The listing builds one solid part. Answer for the finished solid, in the listing's coordinates (mm). A direction names the side the tool comes from. Give positions to 0.01 mm unless a question says otherwise; leave off trailing zeros. Write each loop counter-clockwise with the first axis right and the second up, starting at its lowest first coordinate (ties: lowest second). Pieces come first, ordered by that corner, then holes. Notation, with made-up numbers: (14.25, -37) - (39.25, -37) arc R16 ccw to (39.25, -28) - close; hole circle Ø8 at (36.5, -29). An arc over 180 degrees is marked (long way). Use a Markdown table: item, result. Add a question column.
from build123d import *

# Parameters (mm, degrees)
SKETCH1_R              = 1.5
BOSS_EXTRUDE1_DEPTH    = 3.6
FILLET1_R              = 1.5
LPATTERN2_COUNT        = 6
LPATTERN2_PITCH        = 38.5
FILLET1_OF_LPATTERN2_R = 1.5


with BuildPart() as part:
    # Sketch1 → Boss-Extrude1 (new body)
    with BuildSketch(Plane.XY):
        Polygon((-19.25, 14.2), (-19.25, 0), (-19.25, -20), (19.25, -20), (19.25, 0), (19.25, 14.2), (12, 14.2), (11.5, 4.2), (5, 4.2), (5, 0), (-5, 0), (-5, 4.2), (-11.5, 4.2), (-12, 14.2), align=None)
        with Locations((0, -10)):
            Circle(SKETCH1_R, mode=Mode.SUBTRACT)
    boss_extrude1 = extrude(amount=BOSS_EXTRUDE1_DEPTH)

    # Fillet1
    fillet1_edges = [part.edges().sort_by_distance(p)[0] for p in [
        (-5, 0, 1.8),
        (5, 0, 1.8),
    ]]
    fillet(fillet1_edges, radius=FILLET1_R)

    # LPattern2: Boss-Extrude1 ×6
    with Locations(*[(i * LPATTERN2_PITCH, 0, 0) for i in range(1, LPATTERN2_COUNT)]):
        add(boss_extrude1)

    # Fillet1 of LPattern2
    fillet1_of_lpattern2_edges = [part.edges().sort_by_distance(p)[0] for p in [
        (33.5, 0, 1.8),
        (43.5, 0, 1.8),
        (72, 0, 1.8),
        (82, 0, 1.8),
        (110.5, 0, 1.8),
        (120.5, 0, 1.8),
        (149, 0, 1.8),
        (159, 0, 1.8),
        (187.5, 0, 1.8),
        (197.5, 0, 1.8),
    ]]
    fillet(fillet1_of_lpattern2_edges, radius=FILLET1_OF_LPATTERN2_R)


solid = part.part
1. Consider L1, parallel to Y at x = 77, z = 2.4; L2, parallel to Y at x = 125, z = 2; L3, parallel to Y at x = -2, z = 0.85. Determine where each line is inside the solid, lowest interval first. Write a range as [from, to].
2. The part is cut by section B-B (x = 30). Give the vertices of the cut face in (y, z).
3. Given P1, Ø1.8, axis at x = 38.5, y = -10, coming from the -Z side; P2, Ø1.1, axis at x = 194, z = 2, coming from the +Y side; P3, Ø1.1, axis at x = 46.5, z = 1.5, coming from the +Y side, each flat-ended and moving along its own axis, determine where each tip first touches the part or whether it passes through.
4. For a pull along X with two mould halves and no side action, classify faces 3 (the flat face through (96, 14.2, 2)), 4 (the flat face through (-19.25, -3, 2)), 5 (the flat face through (204.254, 9.27, 1.775)) as released by +X, released by -X, zero draft, split by the parting line, or undercut.
5. Which of the six approach directions +Z, -Z, +X, -X, +Y, -Y give full straight-line access (tool end or side, diameter ignored) to faces 1 (the flat face through (-16, 14.2, 2)), 2 (the flat face through (127.254, 9.27, 1.775))?
6. The part is cut by section A-A (z = 0.9). Count the separate pieces of the cut face and the enclosed holes in it, and give its area (3 significant figures).
Check values:
| question | item | result |
|---|---|---|
| 1 | L1 | y = [-20, -11.5], [-8.5, 0] |
| 1 | L2 | y = [-20, 4.2] |
| 1 | L3 | y = [-20, 0] |
| 2 | outline | (-20, 0) - (4.2, 0) - (4.2, 3.6) - (-20, 3.6) - close |
| 3 | P1 | passes through |
| 3 | P2 | stops at y = 0 |
| 3 | P3 | stops at y = 4.2 |
| 4 | face 3 | zero draft |
| 4 | face 4 | released by -X |
| 4 | face 5 | undercut |
| 5 | face 1 | +Z, -Z, +X, -X, +Y |
| 5 | face 2 | +Z, -Z, +Y |
| 6 | separate pieces | 1 |
| 6 | enclosed holes | 6 |
| 6 | area | 6,200 mm2 |
